Design review of the part built by this model. Coordinates are the model's own, in mm. Give positions to 0.01 mm unless a question says otherwise; leave off trailing zeros. Order: outer loops, then holes, each group sorted by start corner. A loop starts at its lowest first (then second) coordinate and runs counter-clockwise, first axis right, second up. Notation, with made-up numbers: M -34.75,10.25 L -10.75,10.25 A13 ccw -10.75,29.25 Z; hole C 62,19.5 d6. An arc over 180 degrees is marked long. Put each result on its own line as item: value. Start each with the question number.
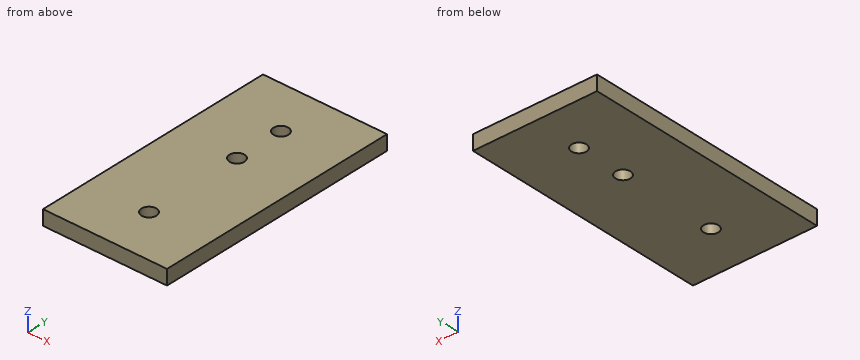
Autodesk Inventor part; units mm, degrees
ref_plane "YZ Plane" through (0, 0, 0) normal (1, 0, 0) x (0, 1, 0)
ref_plane "XZ Plane" through (0, 0, 0) normal (0, 1, 0) x (-1, 0, 0)
ref_plane "XY Plane" through (0, 0, 0) normal (0, 0, 1) x (1, 0, 0)
sketch "Sketch1" plane through (0, 0, 0) normal (0, 0, 1) x (1, 0, 0)
  line L0 (0, 0) -> (25, 0)
  line L1 (25, 0) -> (25, -50)
  line L2 (0, -50) -> (0, 0)
  circle A0 centre (12.5, -40) radius 1.5
  circle A1 centre (12.5, -20) radius 1.5
  circle A2 centre (12.5, -10) radius 1.5
  line L3 (12.5, -50) -> (0, -50)
  line L4 (12.5, -50) -> (25, -50)
  dimension "d6" = 3
  dimension "d7" = 3
extrude "Extrusion1" add sketch "Sketch1" along normal blind 3
properties part number "plat sim"
1. Consider section A-A on z = 2.55. Give the boundary of the cut face in (x, y), then the cut area to 3 significant figures.
2. To check wall thickness, follow probe 1 along Y at (x, z) = (12.5, 1.15); probe 2 along Y at (x, z) = (12, 0.9). State the ranges of each line that lie inside material, in increasing order.
3. Consider section C-C on x = 12.5. Give the boundary of the cut face in (y, z).
4. Insertion check: pin 1 (4 mm diameter, centred on x = 12.5, y = -40, fed in from +Z). The pin has a flat end and moves straight along its axis. Give the tip position at first contact, or say it passes through.
5. Consider section B-B on y = -10. Give the boundary of the cut face in (x, z).
Returned:
1. outline: M 0,-50 L 25,-50 L 25,0 L 0,0 Z; hole C 12.5,-40 d3; hole C 12.5,-20 d3; hole C 12.5,-10 d3
1. area: 1,230 mm2
2. probe 1: y = -50 to -41.5, -38.5 to -21.5, -18.5 to -11.5, -8.5 to 0
2. probe 2: y = -50 to -41.41, -38.59 to -21.41, -18.59 to -11.41, -8.59 to 0
3. outline: M -50,0 L -41.5,0 L -41.5,3 L -50,3 Z; M -38.5,0 L -21.5,0 L -21.5,3 L -38.5,3 Z; M -18.5,0 L -11.5,0 L -11.5,3 L -18.5,3 Z; M -8.5,0 L 0,0 L 0,3 L -8.5,3 Z
4. pin 1: stops at z = 3
5. outline: M 0,0 L 11,0 L 11,3 L 0,3 Z; M 14,0 L 25,0 L 25,3 L 14,3 Z
